Build history of the part. All positions in model axes, mm. A direction names the side the tool comes from. Round coordinates to 2 decimals unless told otherwise and drop trailing zeros. Loops run counter-clockwise (first coordinate to the right, second up) from the corner with the lowest first, then second, coordinate; pieces in that order, holes last. Notation, with made-up numbers: (71.25, -0.75) - (124.25, -0.75) arc R18 cw to (124.25, 4.25) - close; hole circle Ø7 at (-13.75, 21.25). An arc over 180 degrees is marked (long way). Use one line per item in the form item = value. Start each with the question number.
Q1. Saw through at D-D (x = -2.5). Give the cut face in (y, z).
Q2. 3-axis set-ups, long thin cutter, end or side, ignore diameter. For faces 5 (the face through (10, -4, 10)), 6 (the face through (13, -3, -17)), 7 (the face through (3, -3.5, 3)): which of +Z, -Z, +X, -X, +Y, -Y reach the whole face in a straight line?
Q3. Saw through at C-C (x = 10). Give the cut face in (y, z).
Q4. Drill centre lines: line 1 (Z direction, x = 10, y = -1.8); line 2 (Y direction, x = -6.5, z = -6); line 3 (Z direction, x = 12, y = -4.25). Where is each one in solid material? Low to high.
Q5. Saw through at A-A (z = -15). Give the cut face in (x, y).
Q6. Saw through at B-B (y = -0.75). Give the cut face in (x, z).
Q7. Mould opens along Z. For faces 1 (the face through (-5, -6, -5)), 2 (the face through (-17.32, -1.03, 7.87)), 3 (the face through (-5, -2, -30)), 4 (the face through (-17, -2, 20)) say: released by +Z, released by -Z, zero draft, split by the parting line, or undercut.
Q8. Pin check, flat tips, straight feed: pin 1 (12 mm diameter, centred on x = 13, z = 11.5, fed in from +Y); pin 2 (4 mm diameter, centred on x = -15.5, z = 7.5, fed in from -Y); pin 3 (3 mm diameter, centred on x = 9, y = -1, fed in from +Z); pin 4 (5.5 mm diameter, centred on x = -15, z = 10, fed in from +Y). Stop position of each tip, or through.
```python
from build123d import *

# Parameters (mm, degrees)
CYLINDER009_R     = 3.15
CYLINDER009_DEPTH = 10
CYLINDER008_R     = 3.15
CYLINDER008_DEPTH = 10
CYLINDER006_R     = 6.5
CYLINDER006_DEPTH = 10
CYLINDER007_R     = 6.5
CYLINDER007_DEPTH = 10
BOX010_W          = 28
BOX010_H          = 16
BOX010_DEPTH      = 28
BOX008_W          = 50
BOX008_H          = 6
BOX008_DEPTH      = 50
FILLET_R          = 2
CHAMFER014_SIZE   = 20
CHAMFER015_SIZE   = 2
CHAMFER016_SIZE   = 1
BOX007_W          = 7.8
BOX007_H          = 2
BOX007_DEPTH      = 20
CHAMFER010_SIZE   = 1
BOX009_W          = 20
BOX009_H          = 2
BOX009_DEPTH      = 7.8
CHAMFER013_SIZE   = 1


with BuildPart() as cylinder009:
    # Cylinder009 → Cylinder009 (new body)
    with BuildSketch(Plane(origin=(10, -7, -15), x_dir=(1, 0, 0), z_dir=(0, 1, 0))):
        Circle(CYLINDER009_R)
    extrude(amount=CYLINDER009_DEPTH)


with BuildPart() as fusion005:
    # Cylinder008 → Cylinder008 (new body)
    with BuildSketch(Plane(origin=(-15, -7, 10), x_dir=(1, 0, 0), z_dir=(0, 1, 0))):
        Circle(CYLINDER008_R)
    extrude(amount=CYLINDER008_DEPTH)

    # Fusion005: union Cylinder009
    add(cylinder009.part)


with BuildPart() as cylinder006:
    # Cylinder006 → Cylinder006 (new body)
    with BuildSketch(Plane(origin=(10, -16, -15), x_dir=(1, 0, 0), z_dir=(0, 1, 0))):
        Circle(CYLINDER006_R)
    extrude(amount=CYLINDER006_DEPTH)


with BuildPart() as fusion006:
    # Cylinder007 → Cylinder007 (new body)
    with BuildSketch(Plane(origin=(-15, -16, 10), x_dir=(1, 0, 0), z_dir=(0, 1, 0))):
        Circle(CYLINDER007_R)
    extrude(amount=CYLINDER007_DEPTH)

    # Fusion006: union Cylinder006
    add(cylinder006.part)


with BuildPart() as fusion006_1:
    # Fusion006 placement: moved
    add(fusion006.part.moved(Location((0, 3, 0))))


with BuildPart() as cube010:
    # Box010 → Box010 (new body)
    with BuildSketch(Plane(origin=(-7.5, -3.5, -7.5), x_dir=(1, 0, 0), z_dir=(0, 0, 1))):
        with Locations((14, 8)):
            Rectangle(BOX010_W, BOX010_H)
    extrude(amount=BOX010_DEPTH)


with BuildPart() as chamfer016:
    # Box008 → Box008 (new body)
    with BuildSketch(Plane(origin=(-30, -6, -30), x_dir=(1, 0, 0), z_dir=(0, 0, 1))):
        with Locations((25, 3)):
            Rectangle(BOX008_W, BOX008_H)
    extrude(amount=BOX008_DEPTH)

    # Fillet
    fillet_edges = [chamfer016.edges().sort_by_distance(p)[0] for p in [
        (-30, -3, -30),
    ]]
    fillet(fillet_edges, radius=FILLET_R)

    # Chamfer014
    chamfer014_edges = [chamfer016.edges().sort_by_distance(p)[0] for p in [
        (20, -3, 20),
    ]]
    chamfer(chamfer014_edges, length=CHAMFER014_SIZE)

    # Chamfer015
    chamfer015_edges = [chamfer016.edges().sort_by_distance(p)[0] for p in [
        (20, -3, -30),
        (-30, -3, 20),
    ]]
    chamfer(chamfer015_edges, length=CHAMFER015_SIZE)

    # Cut002008002: cut Cube010
    add(cube010.part, mode=Mode.SUBTRACT)

    # Chamfer016
    chamfer016_edges = [chamfer016.edges().sort_by_distance(p)[0] for p in [
        (20, -6, -14),
        (19, -6, -29),
        (10, -6, 10),
        (-5, -6, -30),
        (-14, -6, 20),
        (-29.414214, -6, -29.414214),
        (-29, -6, 19),
        (-30, -6, -5),
    ]]
    chamfer(chamfer016_edges, length=CHAMFER016_SIZE)


with BuildPart() as chamfer010:
    # Box007 → Box007 (new body)
    with BuildSketch(Plane(origin=(-18.9, -1, 0), x_dir=(1, 0, 0), z_dir=(0, 0, 1))):
        with Locations((3.9, 1)):
            Rectangle(BOX007_W, BOX007_H)
    extrude(amount=BOX007_DEPTH)

    # Chamfer010
    chamfer010_edges = [chamfer010.edges().sort_by_distance(p)[0] for p in [
        (-15, 1, 0),
        (-15, 1, 20),
    ]]
    chamfer(chamfer010_edges, length=CHAMFER010_SIZE)


with BuildPart() as top_corner_clip:
    # Box009 → Box009 (new body)
    with BuildSketch(Plane(origin=(0, -1, -18.9), x_dir=(1, 0, 0), z_dir=(0, 0, 1))):
        with Locations((10, 1)):
            Rectangle(BOX009_W, BOX009_H)
    extrude(amount=BOX009_DEPTH)

    # Chamfer013
    chamfer013_edges = [top_corner_clip.edges().sort_by_distance(p)[0] for p in [
        (0, 1, -15),
        (20, 1, -15),
    ]]
    chamfer(chamfer013_edges, length=CHAMFER013_SIZE)

    # Fusion007: union Chamfer010
    add(chamfer010.part)

    # Fusion008: union Chamfer016
    add(chamfer016.part)

    # Cut002008003: cut Fusion006
    add(fusion006_1.part, mode=Mode.SUBTRACT)

    # Cut002008004: cut Fusion005
    add(fusion005.part, mode=Mode.SUBTRACT)


solid = top_corner_clip.part
```
Report:
q1.outline = (-6, -29) - (-5, -30) - (0, -30) - (0, -7.5) - (-3.5, -7.5) - (-3.5, 20) - (-5, 20) - (-6, 19) - close
q2.face_5 = +Z, +X, +Y, -Y
q2.face_6 = -Y
q2.face_7 = +Z, +X, +Y
q3.outline = (-6, -29) - (-5, -30) - (0, -30) - (0, -18.9) - (1, -18.9) - (1, -18.15) - (-3, -18.15) - (-3, -21.5) - (-6, -21.5) - close; (-6, -8.5) - (-3, -8.5) - (-3, -11.85) - (1, -11.85) - (1, -11.1) - (0, -11.1) - (0, -7.5) - (-3.5, -7.5) - (-3.5, 10) - (-5, 10) - (-6, 8.59) - close
q4.line_1 = -30 to -18.15, -11.85 to -7.5
q4.line_2 = -6 to -3.5
q4.line_3 = -30 to -21.18, -8.82 to 8
q5.outline = (-30, -5) - (-29, -6) - (3.5, -6) - (3.5, -3) - (6.85, -3) - (6.85, 1) - (1, 1) - (0, 0) - (-30, 0) - close; (13.15, -3) - (16.5, -3) - (16.5, -6) - (19, -6) - (20, -5) - (20, 0) - (19, 1) - (13.15, 1) - close
q6.outline = (-30, -28) arc R2 ccw to (-28, -30) - (18, -30) - (20, -28) - (20, -7.5) - (-7.5, -7.5) - (-7.5, 20) - (-28, 20) - (-30, 18) - close; hole circle Ø6.3 at (-15, 10); hole circle Ø6.3 at (10, -15)
q7.face_1 = zero draft
q7.face_2 = undercut
q7.face_3 = released by -Z
q7.face_4 = released by +Z
q8.pin_1 = -3.5
q8.pin_2 = -3
q8.pin_3 = -7.5
q8.pin_4 = through
